from build123d import *

# Parameters (mm, degrees)
SKETCH1_R           = 27
BOSS_EXTRUDE1_DEPTH = 15
CUT_EXTRUDE1_START  = -15
CUT_EXTRUDE1_DEPTH  = 15


with BuildPart() as part:
    # Sketch1 → Boss-Extrude1 (new body)
    with BuildSketch(Plane(origin=(0, 0, 0), x_dir=(1, 0, 0), z_dir=(0, 1, 0))):
        with BuildLine():
            ThreePointArc((-31.523820357, 5.499886369), (-32, 0), (-31.523820357, -5.499886369))
            ThreePointArc((-31.523820357, -5.499886369), (-33.916662735, -18.956279365), (-44.393071751, -27.733810979))
            ThreePointArc((-44.393071751, -27.733810979), (-49.143921292, -49.143921292), (-27.733810979, -44.393071751))
            ThreePointArc((-27.733810979, -44.393071751), (-18.956279365, -33.916662735), (-5.499886369, -31.523820357))
            ThreePointArc((-5.499886369, -31.523820357), (0, -32), (5.499886369, -31.523820357))
            ThreePointArc((5.499886369, -31.523820357), (18.956279365, -33.916662735), (27.733810979, -44.393071751))
            ThreePointArc((27.733810979, -44.393071751), (49.143921292, -49.143921292), (44.393071751, -27.733810979))
            ThreePointArc((44.393071751, -27.733810979), (33.916662735, -18.956279365), (31.523820357, -5.499886369))
            ThreePointArc((31.523820357, -5.499886369), (32, 0), (31.523820357, 5.499886369))
            ThreePointArc((31.523820357, 5.499886369), (33.916662735, 18.956279365), (44.393071751, 27.733810979))
            ThreePointArc((44.393071751, 27.733810979), (49.143921292, 49.143921292), (27.733810979, 44.393071751))
            ThreePointArc((27.733810979, 44.393071751), (18.956279365, 33.916662735), (5.499886369, 31.523820357))
            ThreePointArc((5.499886369, 31.523820357), (0, 32), (-5.499886369, 31.523820357))
            ThreePointArc((-5.499886369, 31.523820357), (-18.956279365, 33.916662735), (-27.733810979, 44.393071751))
            ThreePointArc((-27.733810979, 44.393071751), (-49.143921292, 49.143921292), (-44.393071751, 27.733810979))
            ThreePointArc((-44.393071751, 27.733810979), (-33.916662735, 18.956279365), (-31.523820357, 5.499886369))
        make_face()
        with Locations(Location((0, 0, 0), (0, 0, 270))):
            Circle(SKETCH1_R, mode=Mode.SUBTRACT)
    extrude(amount=BOSS_EXTRUDE1_DEPTH)

    # Sketch2 → Cut-Extrude1 (cut)
    with BuildSketch(Plane(origin=(0, 15, 0), x_dir=(1, 0, 0), z_dir=(0, 1, 0)).offset(CUT_EXTRUDE1_START)):
        with BuildLine():
            Line((15.226129133, 22.297196945), (30.292274874, 37.363342686))
            ThreePointArc((30.292274874, 37.363342686), (47.022600949, 47.022600949), (37.363342686, 30.292274874))
            Line((37.363342686, 30.292274874), (22.297196945, 15.226129133))
            ThreePointArc((22.297196945, 15.226129133), (27, 0), (22.297196945, -15.226129133))
            Line((22.297196945, -15.226129133), (37.363342686, -30.292274874))
            ThreePointArc((37.363342686, -30.292274874), (47.022600949, -47.022600949), (30.292274874, -37.363342686))
            Line((30.292274874, -37.363342686), (15.226129133, -22.297196945))
            ThreePointArc((15.226129133, -22.297196945), (0, -27), (-15.226129133, -22.297196945))
            Line((-15.226129133, -22.297196945), (-30.292274874, -37.363342686))
            ThreePointArc((-30.292274874, -37.363342686), (-47.022600949, -47.022600949), (-37.363342686, -30.292274874))
            Line((-37.363342686, -30.292274874), (-22.297196945, -15.226129133))
            ThreePointArc((-22.297196945, -15.226129133), (-27, 0), (-22.297196945, 15.226129133))
            Line((-22.297196945, 15.226129133), (-37.363342686, 30.292274874))
            ThreePointArc((-37.363342686, 30.292274874), (-47.022600949, 47.022600949), (-30.292274874, 37.363342686))
            Line((-30.292274874, 37.363342686), (-15.226129133, 22.297196945))
            ThreePointArc((-15.226129133, 22.297196945), (0, 27), (15.226129133, 22.297196945))
        make_face()
    extrude(amount=CUT_EXTRUDE1_DEPTH, mode=Mode.SUBTRACT)


solid = part.part
Could you check a few things on this model? Use its own coordinates, in mm. A direction names the side the tool comes from. Give positions to 0.01 mm unless a question says otherwise; leave off trailing zeros. Write each loop counter-clockwise with the first axis right and the second up, starting at its lowest first coordinate (ties: lowest second). Pieces come first, ordered by that corner, then holes. Notation, with made-up numbers: (22, -9) -> (50, -9) arc R20 ccw to (50, 13) -> close; hole circle Ø2 at (51.5, 43). An arc over 180 degrees is marked (long way). Answer as a JSON object with one key per item and string values.
Q1. Suppose I cut it at A-A on z = -8. Write out the boundary of the cut face in (x, y).
Taken from the geometry:
{"outline": "(-31.25, 0) -> (-25.79, 0) -> (-25.79, 15) -> (-31.25, 15) -> close; (25.79, 0) -> (31.25, 0) -> (31.25, 15) -> (25.79, 15) -> close"}
Q2. We'd pull the mould along Z, two halves only. Please class faces 1 (the flat face through (-0.2, 15, 27.2)), 2 (the cylindrical face through (19.1, 7.4, -34)), 3 (the cylindrical face through (46.759, 7.395, -47.277)): released by +Z, released by -Z, zero draft, split by the parting line, or undercut.
Taken from the geometry:
{"face 1": "zero draft", "face 2": "released by -Z", "face 3": "undercut"}
Q3. Please list where these lines run through material, in increasing order: L1, parallel to Z at x = -28, y = 2.5; L2, parallel to Z at x = 40.5, y = 1.5; L3, parallel to X at y = 6, z = 1.
Taken from the geometry:
{"L1": "z = -45.07 to -35.07, -20.93 to 20.93, 35.07 to 45.07", "L2": "z = -52.94 to -49.94, -29.97 to -25.82, 25.82 to 29.97, 49.94 to 52.94", "L3": "x = -31.98 to -26.98, 26.98 to 31.98"}
Q4. Suppose I cut it at D-D on x = 43. Write out the boundary of the cut face in (y, z), then the cut area to 3 significant figures.
Taken from the geometry:
{"outline": "(0, -52.59) -> (15, -52.59) -> (15, -49.48) -> (0, -49.48) -> close; (0, -30.43) -> (15, -30.43) -> (15, -27.17) -> (0, -27.17) -> close; (0, 27.17) -> (15, 27.17) -> (15, 30.43) -> (0, 30.43) -> close; (0, 49.48) -> (15, 49.48) -> (15, 52.59) -> (0, 52.59) -> close", "area": "191 mm²"}
Q5. Suppose I cut it at C-C on z = -43. Write out the boundary of the cut face in (x, y).
Taken from the geometry:
{"outline": "(-52.59, 0) -> (-49.48, 0) -> (-49.48, 15) -> (-52.59, 15) -> close; (-30.43, 0) -> (-27.17, 0) -> (-27.17, 15) -> (-30.43, 15) -> close; (27.17, 0) -> (30.43, 0) -> (30.43, 15) -> (27.17, 15) -> close; (49.48, 0) -> (52.59, 0) -> (52.59, 15) -> (49.48, 15) -> close"}
Q6. Which directions (+Z, -Z, +X, -X, +Y, -Y) give clear straight access to the entire face, cutting with the end or side of a thin tool? Please do faces 4 (the flat face through (-22.65, 7.4, 29.72)), 5 (the flat face through (-0.2, 0, 27.2)).
Taken from the geometry:
{"face 4": "+Y, -Y", "face 5": "+Z, -Z, +X, -X, -Y"}
Q7. Will these pins go through, and if not, where does the flat tip stop? pin 1 Ø4 at (x, y) = (-25, 5.5) entering from +Z; pin 2 Ø3 at (y, z) = (9.5, -11) entering from -X; pin 3 Ø1.5 at (y, z) = (11.5, -23) entering from +X.
Taken from the geometry:
{"pin 1": "stops at z = 42.64", "pin 2": "stops at x = -31.55", "pin 3": "stops at x = 37.79"}
